Verification items for the finished model (mm, model axes). A direction names the side the tool comes from. Round coordinates to 2 decimals unless told otherwise and drop trailing zeros. Loops run counter-clockwise (first coordinate to the right, second up) from the corner with the lowest first, then second, coordinate; pieces in that order, holes last. Notation, with made-up numbers: (23, 77.5) -> (46, 77.5) arc R23 ccw to (46, 111.5) -> close; hole circle Ø6 at (30.5, 61.25). An arc over 180 degrees is marked (long way). Write item = value, one per line.
```python
from build123d import *

# Parameters (mm, degrees)
SKETCH_2_R      = 1.5
SKETCH_2_R_2    = 0.8
SKETCH_2_R_3    = 2.66
EXTRUDE_1_DEPTH = 1.5


with BuildPart() as part:
    # 草图2 → 凸台-拉伸1 (new body)
    with BuildSketch(Plane.XY):
        with BuildLine():
            Line((5.188427748, -15.986660076), (44, -15.986660076))
            Line((44, -15.986660076), (44, -22))
            Line((44, -22), (5.196152423, -22))
            ThreePointArc((5.196152423, -22), (0, -25), (-5.196152423, -22))
            Line((-5.196152423, -22), (-44, -22))
            Line((-44, -22), (-44, -15.986660076))
            Line((-44, -15.986660076), (-5.188427748, -15.986660076))
            ThreePointArc((-5.188427748, -15.986660076), (0, -13), (5.188427748, -15.986660076))
        make_face()
        with Locations((41, -19)):
            Circle(SKETCH_2_R, mode=Mode.SUBTRACT)
        with Locations((-41, -19)):
            Circle(SKETCH_2_R, mode=Mode.SUBTRACT)
        with Locations((4.25, -19)):
            Circle(SKETCH_2_R_2, mode=Mode.SUBTRACT)
        with Locations((-4.25, -19)):
            Circle(SKETCH_2_R_2, mode=Mode.SUBTRACT)
        with Locations((0, -14.75)):
            Circle(SKETCH_2_R_2, mode=Mode.SUBTRACT)
        with Locations((0, -23.25)):
            Circle(SKETCH_2_R_2, mode=Mode.SUBTRACT)
        with Locations((0, -19)):
            Circle(SKETCH_2_R_3, mode=Mode.SUBTRACT)
        with Locations((-18.8, -19)):
            Circle(SKETCH_2_R, mode=Mode.SUBTRACT)
        with Locations((18.8, -19)):
            Circle(SKETCH_2_R, mode=Mode.SUBTRACT)
    extrude(amount=EXTRUDE_1_DEPTH)


solid = part.part
```
(1) Sectioned sample at D-D, the plane y = -14.75. Record the cut outline in (x, z), and give its area (3 significant figures).
Filled sheet:
outline = (-4.24, 0) -> (-0.8, 0) -> (-0.8, 1.5) -> (-4.24, 1.5) -> close; (0.8, 0) -> (4.24, 0) -> (4.24, 1.5) -> (0.8, 1.5) -> close
area = 10.3 mm2
(2) Draft check along X on faces 1 (the face through (18.605, -17.513, 0.74)), 2 (the face through (44, -19, 1)), 3 (the face through (25, -22, 1)). Enter one of: released by +X, released by -X, zero draft, split by the parting line, or undercut.
Filled sheet:
face_1 = undercut
face_2 = released by +X
face_3 = zero draft
(3) Set-up check for faces 4 (the face through (-25, -15.987, 1)), 5 (the face through (-24, -22, 1)), 6 (the face through (24, -15.987, 1)): record each of +Z, -Z, +X, -X, +Y, -Y from which the full face is reachable in a straight line by a thin tool's end or side.
Filled sheet:
face_4 = +Z, -Z, -X, +Y
face_5 = +Z, -Z, -X, -Y
face_6 = +Z, -Z, +X, +Y
(4) Material ranges on probe 1 along Y at (x, z) = (18.8, 1.1); probe 2 along Y at (x, z) = (15, 1.05); probe 3 along X at (y, z) = (-16.75, 1.35), recorded low to high. Write a range as from..to.
Filled sheet:
probe_1 = -22..-20.5, -17.5..-15.99
probe_2 = -22..-15.99
probe_3 = -44..-1.42, 1.42..44
(5) Sectioned sample at B-B, the plane z = 1.05. Count the separate pieces of the cut face and the enclosed holes in it, and give its area (3 significant figures).
Filled sheet:
separate_pieces = 1
enclosed_holes = 9
area = 515 mm2
(6) Sectioned sample at C-C, the plane x = 0. Record the cut outline in (y, z), and give its area (3 significant figures).
Filled sheet:
outline = (-25, 0) -> (-24.05, 0) -> (-24.05, 1.5) -> (-25, 1.5) -> close; (-22.45, 0) -> (-21.66, 0) -> (-21.66, 1.5) -> (-22.45, 1.5) -> close; (-16.34, 0) -> (-15.55, 0) -> (-15.55, 1.5) -> (-16.34, 1.5) -> close; (-13.95, 0) -> (-13, 0) -> (-13, 1.5) -> (-13.95, 1.5) -> close
area = 5.22 mm2
(7) Go/stop test with flat-tipped pins: pin 1 Ø5 at (x, y) = (-41, -19) entering from -Z; pin 2 Ø0.8 at (x, z) = (-17, 1) entering from +Y. Record where each tip stops, or that it passes through.
Filled sheet:
pin_1 = 0
pin_2 = -15.99
(8) Sectioned sample at A-A, the plane x = -18.8. Record the cut outline in (y, z), and give its area (3 significant figures).
Filled sheet:
outline = (-22, 0) -> (-20.5, 0) -> (-20.5, 1.5) -> (-22, 1.5) -> close; (-17.5, 0) -> (-15.99, 0) -> (-15.99, 1.5) -> (-17.5, 1.5) -> close
area = 4.52 mm2
